CAD build for the part. Positions are in the model's coordinates, mm. A direction names the side the tool comes from. Give positions to 0.01 mm unless a question says otherwise; leave off trailing zeros. Write each loop counter-clockwise with the first axis right and the second up, starting at its lowest first coordinate (ties: lowest second). Pieces come first, ordered by that corner, then holes. Notation, with made-up numbers: (2, 61.25) - (14, 61.25) arc R25 cw to (14, 80.25) - close; hole circle Ø7 at (39, -33.75). An arc over 180 degrees is marked (long way). Answer as a JSON object with one key per item and string values.
Autodesk Fusion 360 part; units mm, degrees
sketch "Sketch1" plane through (0, 0, 0) normal (0, 1, 0) x (1, 0, 0)
  line L0 (29.7004, -65.6) -> (29.7004, -55.6)
  line L1 (29.7004, -55.6) -> (9.7004, -55.6)
  line L2 (9.7004, -55.6) -> (9.7004, -25)
  line L3 (9.7004, -25) -> (29.7004, -25)
  line L4 (29.7004, -25) -> (29.7004, -15)
  line L5 (29.7004, -15) -> (-0.2996, -15)
  line L6 (-0.2996, -15) -> (-0.2996, -65.6)
  line L7 (-0.2996, -65.6) -> (29.7004, -65.6)
  dimension "d1" = 10
  dimension "d2" = 10
  dimension "d5" = 10
  dimension "d6" = 30
  dimension "d7" = 50.6
  dimension "d8" = 30
extrude "Extrude1" add sketch "Sketch1" along normal blind 40
sketch "Sketch2" plane through (0, 0, 15) normal (0, 0, -1) x (1, 0, 0)
  line L0 (29.7004, 0) -> (-0.2996, 0)
  line L1 (-0.2996, 0) -> (-0.2996, -40)
  line L2 (-0.2996, -40) -> (29.7004, -40)
  line L3 (29.7004, -40) -> (29.7004, 0)
  circle A0 centre (29.7004, -20) radius 20
  circle A1 centre (29.7004, -20) radius 10
  dimension "d11" = 20
extrude "Extrude2" add sketch "Sketch2" against normal blind 10 contours L3 A0 A1 picked at (46.2992, -20.9488)
extrude "Extrude3" cut sketch "Sketch2" against normal blind 10 contours L3 A1 picked at (35.3898, -22.165)
fillet "Fillet1" radius 10 1 edges at (-0.2996, 20, 15)
fillet "Fillet2" radius 10 1 edges at (9.7004, 20, 25)
fillet "Fillet3" radius 10 2 edges at (29.7004, 0, 60.6) (29.7004, 40, 60.6)
(1) Saw through at C-C, the plane z = 60. Give the cut face in (x, y), and give its area (3 significant figures).
Answer key:
{"outline": "(-0.3, 0) - (19.7, 0) arc R10 ccw to (29.7, 10) - (29.7, 30) arc R10 ccw to (19.7, 40) - (-0.3, 40) - close", "area": "1,160 mm²"}
(2) 3-axis set-ups, long thin cutter, end or side, ignore diameter. For faces 1 (the face through (26.69, 37.15, 60.53)), 2 (the face through (26.85, 3.01, 60.53)), 3 (the face through (29.7, 20, 20)), 4 (the face through (9.7, 20, 45)): which of +Z, -Z, +X, -X, +Y, -Y reach the whole face in a straight line?
Answer key:
{"face 1": "+Z, +X, +Y", "face 2": "+Z, +X, -Y", "face 3": "+Z, -Z", "face 4": "+X, +Y, -Y"}
(3) Flat gauge pins, fed straight in: P1, Ø16.5, axis at y = 28.5, z = 50, coming from the +X side; P2, Ø5, axis at y = 22.5, z = 17.5, coming from the +X side. Where does each tip first touch, or does it go through?
Answer key:
{"P1": "stops at x = 29.7", "P2": "stops at x = 49.7"}
(4) Saw through at A-A, the plane y = 20. Give the cut face in (x, z).
Answer key:
{"outline": "(-0.3, 25) arc R10 ccw to (9.7, 15) - (29.7, 15) - (29.7, 25) - (19.7, 25) arc R10 cw to (9.7, 35) - (9.7, 55.6) - (29.7, 55.6) - (29.7, 65.6) - (-0.3, 65.6) - close; (39.7, 15) - (49.7, 15) - (49.7, 25) - (39.7, 25) - close"}
(5) Saw through at B-B, the plane x = 28. Give the cut face in (y, z), and give its area (3 significant figures).
Answer key:
{"outline": "(0, 15) - (40, 15) - (40, 25) - (0, 25) - close; (4.42, 55.6) - (35.58, 55.6) - (35.58, 65.6) - (4.42, 65.6) - close", "area": "712 mm²"}
(6) Pull direction X, two halves, no side cores. Call faces 5 (the face through (39.7, 20.2, 19.9)), 6 (the face through (28, 20, 25)), 7 (the face through (29.7, 20, 61)): pulls with the +X half, pulls with the -X half, needs draft (parallel to the pull), parting line crosses it, or undercut.
Answer key:
{"face 5": "undercut", "face 6": "needs draft", "face 7": "pulls with the +X half"}
(7) Saw through at D-D, the plane y = 28. Give the cut face in (x, z).
Answer key:
{"outline": "(-0.3, 25) arc R10 ccw to (9.7, 15) - (29.7, 15) - (29.7, 25) - (19.7, 25) arc R10 cw to (9.7, 35) - (9.7, 55.6) - (29.7, 55.6) - (29.7, 65.6) - (-0.3, 65.6) - close; (35.7, 15) - (48.03, 15) - (48.03, 25) - (35.7, 25) - close"}
(8) Probe L1, parallel to X at y = 26.5, z = 41.5; L2, parallel to Y at x = 36.5, z = 19.5; L3, parallel to Z at x = 18, y = 6.5. List the from-to ranges inside material, lowest first. Write a range as [from, to].
Answer key:
{"L1": "x = [-0.3, 9.7]", "L2": "y = [1.19, 12.67], [27.33, 38.81]", "L3": "z = [15, 25.15], [55.6, 65.6]"}
